Source: CAD feature listing. Evaluate the final solid. Frame: model axes, mm. A direction names the side the tool comes from. Coordinates: 2 decimals unless noted, no trailing zeros. Loops run counter-clockwise (first coordinate to the right, second up) from the corner with the lowest first, then second, coordinate; pieces in that order, holes last.
Item 1: Reachability of faces 5 (the flat face through (0, 6, 29.285)), 6 (the flat face through (0, 6, 32.185)) from +Z, -Z, +X, -X, +Y, -Y: full face, straight path, thin tool, end or side. Return the list, or none.
Item 2: Section query B-B, the plane x = 6. Return the cut outline in (y, z) (3 decimals).
Item 3: Pin query (flat end, axial travel): pin 1 Ø6 at (y, z) = (9, -22.5) entering from -X; pin 2 Ø1.5 at (y, z) = (5.5, -2) entering from +X. Return the tip coordinate at first contact, or that it passes through.
Item 4: Pull-direction query (Y, two-part tool) for faces 1 (the flat face through (0, 2.9, 0)), 2 (the flat face through (-1, 11.5, 0)), 3 (the flat face through (0, 8.6, 0)), 4 (the flat face through (28, 1.2, 0.1)); classes: +Y half, -Y half, draft (parallel to the pull), parting line (faces both ways), or undercut.
Item 5: Section query C-C, the plane y = 3.75. Return the cut outline in (x, z) (3 decimals).
Item 6: Section query A-A, the plane z = -2. Return the cut outline in (x, y).
Item 7: Line query: probe 1 along Y at (x, z) = (-10, 15); probe 2 along Z at (x, y) = (-12, 7.25) (3 decimals); probe 3 along X at (y, z) = (9.5, 23). Output: solid intervals per line, ascending.
```python
from build123d import *

# Parameters (mm, degrees)
SKETCH1_W           = 56
SKETCH1_H           = 64.37
SKETCH1_W_2         = 50
SKETCH1_H_2         = 58.37
BOSS_EXTRUDE1_DEPTH = 11.5
SKETCH2_W           = 58.57
SKETCH2_H           = 5.7
CUT_EXTRUDE1_DEPTH  = 103
FILLET1_R           = 1


with BuildPart() as part:
    # Sketch1 → Boss-Extrude1 (new body)
    # profile 1 of 2: a face of its own
    with BuildSketch(Plane(origin=(0, 0, 0), x_dir=(1, 0, 0), z_dir=(0, 1, 0))):
        Rectangle(SKETCH1_W, SKETCH1_H)
        Rectangle(SKETCH1_W_2, SKETCH1_H_2, mode=Mode.SUBTRACT)
    # profile 2 of 2: a face of its own
    with BuildSketch(Plane(origin=(0, 0, 0), x_dir=(1, 0, 0), z_dir=(0, 1, 0))):
        Rectangle(SKETCH1_W_2, SKETCH1_H_2)
    extrude(amount=BOSS_EXTRUDE1_DEPTH)

    # Sketch2 → Cut-Extrude1 (cut)
    with BuildSketch(Plane.ZY.offset(28)):
        with Locations((0, 5.75)):
            Rectangle(SKETCH2_W, SKETCH2_H)
    extrude(amount=-CUT_EXTRUDE1_DEPTH, mode=Mode.SUBTRACT)

    # Fillet1
    fillet1_edges = [part.edges().sort_by_distance(p)[0] for p in [
        (0, 11.5, 32.185),
        (28, 11.5, 0),
        (0, 11.5, -32.185),
        (28, 2.9, 0),
        (-28, 5.75, -29.285),
        (-28, 8.6, 0),
        (28, 5.75, 29.285),
        (28, 5.75, -29.285),
        (28, 8.6, 0),
        (-28, 2.9, 0),
        (-28, 5.75, 29.285),
        (0, 0, -32.185),
        (28, 0, 0),
        (0, 0, 32.185),
        (-28, 0, 0),
        (-28, 5.75, -32.185),
        (28, 5.75, -32.185),
        (28, 5.75, 32.185),
        (-28, 5.75, 32.185),
    ]]
    fillet(fillet1_edges, radius=FILLET1_R)


solid = part.part
```
Verdict:
1. face 5: +X, -X
1. face 6: +Z, +X, -X, +Y, -Y
2. outline: (0, -31.185) arc R1 ccw to (1, -32.185) - (10.5, -32.185) arc R1 ccw to (11.5, -31.185) - (11.5, 31.185) arc R1 ccw to (10.5, 32.185) - (1, 32.185) arc R1 ccw to (0, 31.185) - close; hole (2.9, -29.285) - (8.6, -29.285) - (8.6, 29.285) - (2.9, 29.285) - close
3. pin 1: stops at x = -28
3. pin 2: passes through
4. face 1: undercut
4. face 2: +Y half
4. face 3: undercut
4. face 4: draft
5. outline: (-28, -31.185) arc R1 ccw to (-27, -32.185) - (27, -32.185) arc R1 ccw to (28, -31.185) - (28, -30.285) arc R1 ccw to (27, -29.285) - (-27, -29.285) arc R1 ccw to (-28, -30.285) - close; (-28, 30.285) arc R1 ccw to (-27, 29.285) - (27, 29.285) arc R1 ccw to (28, 30.285) - (28, 31.185) arc R1 ccw to (27, 32.185) - (-27, 32.185) arc R1 ccw to (-28, 31.185) - close
6. outline: (-28, 1) arc R1 ccw to (-27, 0) - (27, 0) arc R1 ccw to (28, 1) - (28, 1.9) arc R1 ccw to (27, 2.9) - (-27, 2.9) arc R1 ccw to (-28, 1.9) - close; (-28, 9.6) arc R1 ccw to (-27, 8.6) - (27, 8.6) arc R1 ccw to (28, 9.6) - (28, 10.5) arc R1 ccw to (27, 11.5) - (-28, 11.5) - close
7. probe 1: y = 0 to 2.9, 8.6 to 11.5
7. probe 2: z = -32.185 to -29.285, 29.285 to 32.185
7. probe 3: x = -27.99 to 27.99
